Verification items for the finished model (mm, model axes). Give positions to 0.01 mm unless a question says otherwise; leave off trailing zeros. Write each loop counter-clockwise with the first axis right and the second up, starting at its lowest first coordinate (ties: lowest second). Pieces come first, ordered by that corner, then holes.
from build123d import *

# Parameters (mm, degrees)
F0_W     = 110
F0_H     = 70
F1_DEPTH = 5
F2_W     = 20
F2_H     = 8
F3_DEPTH = 5.001
F4_R     = 2.5
F5_DEPTH = 5.001
F6_R     = 2.5
F7_DEPTH = 5.001


with BuildPart() as f1:
    # F0 (on Top) → F1 (new body)
    with BuildSketch(Plane.XY):
        Rectangle(F0_W, F0_H)
    extrude(amount=F1_DEPTH)

    # F2 (on face) → F3 (cut, through all)
    with BuildSketch(Plane.XY.offset(5)):
        Rectangle(F2_W, F2_H)
    extrude(amount=-F3_DEPTH, mode=Mode.SUBTRACT)

    # F4 (on face) → F5 (cut, through all)
    with BuildSketch(Plane.XY.offset(5)):
        with Locations((-25.5, 0)):
            Circle(F4_R)
    extrude(amount=-F5_DEPTH, mode=Mode.SUBTRACT)

    # F6 (on face) → F7 (cut, through all)
    with BuildSketch(Plane.XY.offset(5)):
        with Locations((25.5, 0)):
            Circle(F6_R)
    extrude(amount=-F7_DEPTH, mode=Mode.SUBTRACT)


solid = f1.part
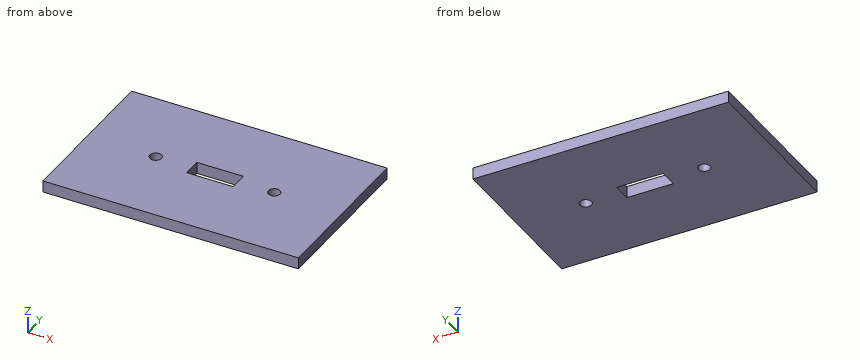
Item 1: Sectioned sample at C-C on y = 0. Record the cut outline in (x, z).
Answer key:
outline: (-55, 0) - (-28, 0) - (-28, 5) - (-55, 5) - close; (-23, 0) - (-10, 0) - (-10, 5) - (-23, 5) - close; (10, 0) - (23, 0) - (23, 5) - (10, 5) - close; (28, 0) - (55, 0) - (55, 5) - (28, 5) - close
Item 2: Sectioned sample at D-D on x = 4.5. Record the cut outline in (y, z).
Answer key:
outline: (-35, 0) - (-4, 0) - (-4, 5) - (-35, 5) - close; (4, 0) - (35, 0) - (35, 5) - (4, 5) - close
Item 3: Scan lines: line 1 along Y through (x, z) = (25.5, 3.15); line 2 along Y through (x, z) = (9.5, 1.65). Record each from-to range of solid material in increasing order.
Answer key:
line 1: y = -35 to -2.5, 2.5 to 35
line 2: y = -35 to -4, 4 to 35
Item 4: Sectioned sample at A-A on x = 25.5. Record the cut outline in (y, z).
Answer key:
outline: (-35, 0) - (-2.5, 0) - (-2.5, 5) - (-35, 5) - close; (2.5, 0) - (35, 0) - (35, 5) - (2.5, 5) - close
Item 5: Sectioned sample at B-B on z = 4.1. Record the cut outline in (x, y).
Answer key:
outline: (-55, -35) - (55, -35) - (55, 35) - (-55, 35) - close; hole circle Ø5 at (-25.5, 0); hole (-10, -4) - (10, -4) - (10, 4) - (-10, 4) - close; hole circle Ø5 at (25.5, 0)
